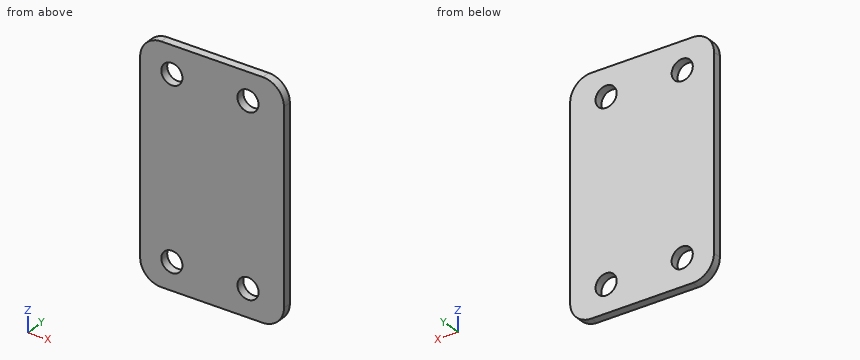
from build123d import *

# Parameters (mm, degrees)
SKETCH1_W           = 40
SKETCH1_H           = 55
BOSS_EXTRUDE1_DEPTH = 2
SKETCH3_R           = 2.5
CUT_EXTRUDE1_DEPTH  = 2
SKETCH4_W           = 6
SKETCH4_H           = 55
CUT_EXTRUDE2_DEPTH  = 2
FILLET1_R           = 5


with BuildPart() as part:
    # Sketch1 → Boss-Extrude1 (new body)
    with BuildSketch(Plane(origin=(0, 0, 0), x_dir=(1, 0, 0), z_dir=(0, 1, 0))):
        Rectangle(SKETCH1_W, SKETCH1_H)
    extrude(amount=BOSS_EXTRUDE1_DEPTH)

    # Sketch3 → Cut-Extrude1 (cut)
    with BuildSketch(Plane(origin=(0, 2, 0), x_dir=(1, 0, 0), z_dir=(0, 1, 0))):
        with Locations((-12.5, 21)):
            Circle(SKETCH3_R)
        with Locations((-12.5, -21)):
            Circle(SKETCH3_R)
        with Locations((5.5, 21)):
            Circle(SKETCH3_R)
        with Locations((5.5, -21)):
            Circle(SKETCH3_R)
    extrude(amount=-CUT_EXTRUDE1_DEPTH, mode=Mode.SUBTRACT)

    # Sketch4 → Cut-Extrude2 (cut)
    with BuildSketch(Plane(origin=(0, 2, 0), x_dir=(1, 0, 0), z_dir=(0, 1, 0))):
        with Locations((17, 0)):
            Rectangle(SKETCH4_W, SKETCH4_H)
    extrude(amount=-CUT_EXTRUDE2_DEPTH, mode=Mode.SUBTRACT)

    # Fillet1
    fillet1_edges = [part.edges().sort_by_distance(p)[0] for p in [
        (14, 1, 27.5),
        (14, 1, -27.5),
        (-20, 1, -27.5),
        (-20, 1, 27.5),
    ]]
    fillet(fillet1_edges, radius=FILLET1_R)


solid = part.part
Part model, mm, in its own coordinate system. Give positions to 0.01 mm unless a question says otherwise; leave off trailing zeros. Write each loop counter-clockwise with the first axis right and the second up, starting at its lowest first coordinate (ties: lowest second). Pieces come first, ordered by that corner, then holes.
1) Cut at A-A on x = -12.5. Write the cut outline in (y, z).
Resolved:
outline: (0, -27.5) - (2, -27.5) - (2, -23.5) - (0, -23.5) - close; (0, -18.5) - (2, -18.5) - (2, 18.5) - (0, 18.5) - close; (0, 23.5) - (2, 23.5) - (2, 27.5) - (0, 27.5) - close
2) Cut at B-B on z = -21. Write the cut outline in (x, y), then the cut area to 3 significant figures.
Resolved:
outline: (-20, 0) - (-15, 0) - (-15, 2) - (-20, 2) - close; (-10, 0) - (3, 0) - (3, 2) - (-10, 2) - close; (8, 0) - (14, 0) - (14, 2) - (8, 2) - close
area: 48.0 mm2
3) Probe L1, parallel to Z at x = 5.5, y = 0.95; L2, parallel to X at y = 0.7, z = 21; L3, parallel to Z at x = -14.5, y = 1.25. List the from-to ranges inside material, lowest first.
Resolved:
L1: z = -27.5 to -23.5, -18.5 to 18.5, 23.5 to 27.5
L2: x = -20 to -15, -10 to 3, 8 to 14
L3: z = -27.5 to -22.5, -19.5 to 19.5, 22.5 to 27.5
4) Pin check, flat tip, straight feed: pin 1 (6.5 mm diameter, centred on x = 5.5, z = 21, fed in from -Y). Stop position of the tip, or through.
Resolved:
pin 1: stops at y = 0
5) Cut at C-C on y = 0.35. Write the cut outline in (x, z), then the cut area to 3 significant figures.
Resolved:
outline: (-20, -22.5) arc R5 ccw to (-15, -27.5) - (9, -27.5) arc R5 ccw to (14, -22.5) - (14, 22.5) arc R5 ccw to (9, 27.5) - (-15, 27.5) arc R5 ccw to (-20, 22.5) - close; hole circle Ø5 at (-12.5, -21); hole circle Ø5 at (-12.5, 21); hole circle Ø5 at (5.5, -21); hole circle Ø5 at (5.5, 21)
area: 1,770 mm2
